For this review, use the dimensioned drawing (mm, ordinates from the lowest corner) and the shaded views. Give positions to 0.01 mm unless a question says otherwise; leave off trailing zeros. Loops run counter-clockwise (first coordinate to the right, second up) from the corner with the lowest first, then second, coordinate; pieces in that order, holes last. Notation, with made-up numbers: M 86,85 L 112,85 A24 cw 112,119 Z; hole C 32,76 d7. An arc over 180 degrees is marked long. Use one line per item in the form item = value. Start each with the question number.
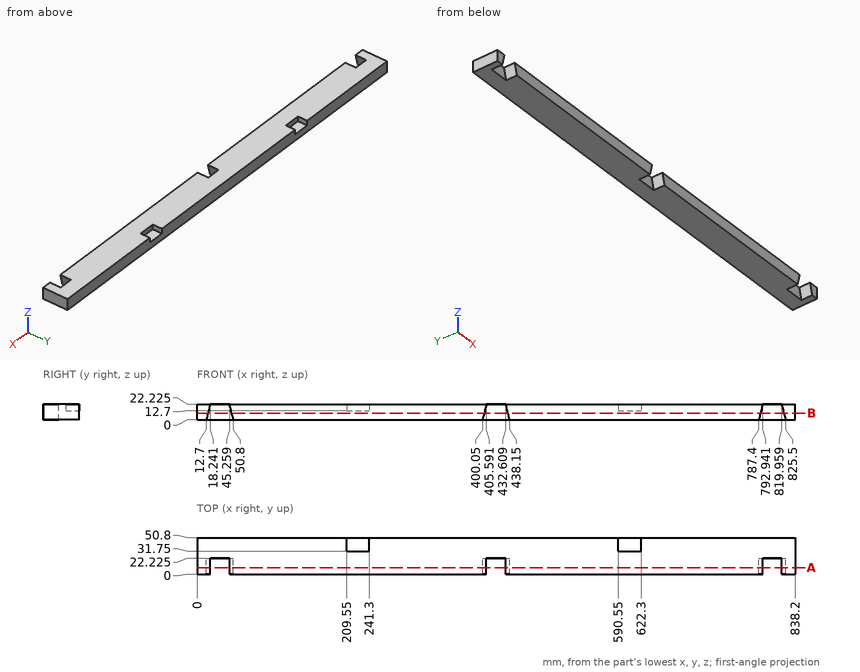
Q1. Take a section at B-B on z = 9.25. Give the boundary of the cut face in (x, y) (1 decimal).
Q2. Wall thickness on probe 1 along X at (y, z) = (42.5, 21.25); probe 2 along X at (y, z) = (20, 3.75) (1 decimal); probe 3 along X at (y, z) = (8, 16.75): over which ranges is each line inside the solid? List them lowest first.
Q3. Clearance check with flat-ended pins moving along their axes: pin 1 Ø5.5 at (x, y) = (232, 40.5) entering from +Z; pin 2 Ø3 at (x, z) = (606.5, 18.5) entering from +Y; pin 3 Ø6.5 at (x, z) = (799, 15) entering from -Y (3 decimals). State where each tip first meets the part, or that it passes through.
Q4. Take a section at A-A on y = 9. State how many separate pieces and enclosed holes the cut face has, plus the area to 3 significant figures.
Response values:
q1.outline = M 0,0 L 15,0 L 15,22.2 L 48.5,22.2 L 48.5,0 L 402.4,0 L 402.4,22.2 L 435.8,22.2 L 435.8,0 L 789.7,0 L 789.7,22.2 L 823.2,22.2 L 823.2,0 L 838.2,0 L 838.2,50.8 L 0,50.8 Z
q2.probe_1 = 0 to 209.55, 241.3 to 590.55, 622.3 to 838.2
q2.probe_2 = 0 to 13.6, 49.9 to 401, 437.2 to 788.3, 824.6 to 838.2
q2.probe_3 = 0 to 16.88, 46.62 to 404.23, 433.97 to 791.58, 821.32 to 838.2
q3.pin_1 = 12.7
q3.pin_2 = 31.75
q3.pin_3 = 22.225
q4.separate_pieces = 4
q4.enclosed_holes = 0
q4.area = 16,500 mm^2
